Verification items for the finished model (mm, model axes). Face numbers are marked on the shaded views. A direction names the side the tool comes from. Round coordinates to 2 decimals unless told otherwise and drop trailing zeros. Write each loop counter-clockwise with the first axis right and the second up, starting at its lowest first coordinate (ties: lowest second). Pieces come first, ordered by that corner, then holes.
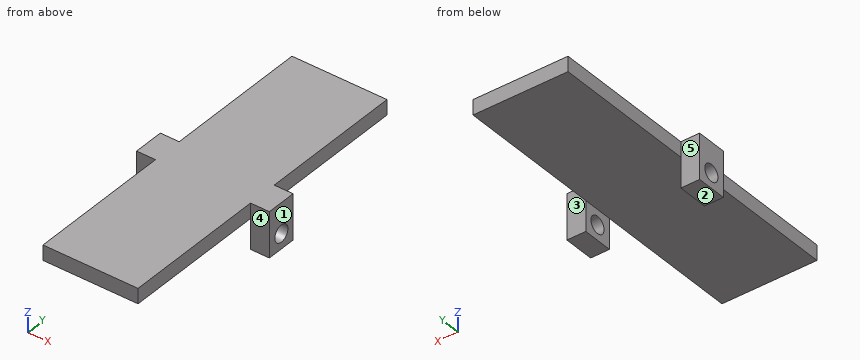
from build123d import *

# Parameters (mm, degrees)
SKETCH1_W           = 16
SKETCH1_H           = 54.011330832
BOSS_EXTRUDE1_DEPTH = 2.54
SKETCH2_W           = 7.62
SKETCH2_H           = 5.141453329
SKETCH2_R           = 1.4224
BOSS_EXTRUDE2_DEPTH = 3.175


with BuildPart() as part:
    # Sketch1 → Boss-Extrude1 (new body)
    with BuildSketch(Plane.XY):
        with Locations((-8, 27.005665416)):
            Rectangle(SKETCH1_W, SKETCH1_H)
    extrude(amount=BOSS_EXTRUDE1_DEPTH)

    # Sketch2 → Boss-Extrude2 (add)
    with BuildSketch(Plane(origin=(0, 0, 0), x_dir=(0, 0, -1), z_dir=(1, 0, 0))):
        with Locations((1.27, 26.974938752)):
            Rectangle(SKETCH2_W, SKETCH2_H)
        with Locations((2.54, 27.005665416)):
            Circle(SKETCH2_R, mode=Mode.SUBTRACT)
    boss_extrude2 = extrude(amount=BOSS_EXTRUDE2_DEPTH)

    # Mirror1: Boss-Extrude2 across plane
    add(boss_extrude2.mirror(Plane.ZY.offset(8)))


solid = part.part
Q1. Sectioned sample at A-A (z = -2.54). Enter the section's corners in (x, y) (3 decimals), plus the area to 3 significant figures.
Recorded:
outline: (-19.175, 24.404) - (-16, 24.404) - (-16, 25.583) - (-19.175, 25.583) - close; (-19.175, 28.428) - (-16, 28.428) - (-16, 29.546) - (-19.175, 29.546) - close; (0, 24.404) - (3.175, 24.404) - (3.175, 25.583) - (0, 25.583) - close; (0, 28.428) - (3.175, 28.428) - (3.175, 29.546) - (0, 29.546) - close
area: 14.6 mm2
Q2. Sectioned sample at C-C (x = -17.5). Enter the section's corners in (y, z), plus the area to 3 significant figures.
Recorded:
outline: (24.4, -5.08) - (29.55, -5.08) - (29.55, 2.54) - (24.4, 2.54) - close; hole circle Ø2.84 at (27.01, -2.54)
area: 32.8 mm2
Q3. Depth check by flat-ended pin: P1, Ø1, axis at x = 1, z = -1.5, coming from the -Y side; P2, Ø3, axis at y = 19, z = -1, coming from the +X side; P3, Ø2.5, axis at x = -18, z = 0, coming from the +Y side; P4, Ø2, axis at y = 44.5, z = -1.5, coming from the -X side. Enter the tip coordinate at first touch or a pass-through.
Recorded:
P1: stops at y = 24.4
P2: stops at x = 0
P3: stops at y = 29.55
P4: passes through
Q4. Sectioned sample at B-B (z = 1.5). Enter the section's corners in (x, y) (3 decimals), plus the area to 3 significant figures.
Recorded:
outline: (-19.175, 24.404) - (-16, 24.404) - (-16, 0) - (0, 0) - (0, 24.404) - (3.175, 24.404) - (3.175, 29.546) - (0, 29.546) - (0, 54.011) - (-16, 54.011) - (-16, 29.546) - (-19.175, 29.546) - close
area: 897 mm2
Q5. Sectioned sample at D-D (y = 42). Enter the section's corners in (x, z).
Recorded:
outline: (-16, 0) - (0, 0) - (0, 2.54) - (-16, 2.54) - close
Q6. Material ranges on line 1 along Y through (x, z) = (-17.3, -2.54); line 2 along X through (y, z) = (24.5, -1) (3 decimals); line 3 along Y through (x, z) = (-17, 2), recorded low to high.
Recorded:
line 1: y = 24.4 to 25.58, 28.43 to 29.55
line 2: x = -19.175 to -16, 0 to 3.175
line 3: y = 24.4 to 29.55
Q7. Tool access check on the marked faces 1, 2, 3, 4 and 5. Record the directions out of +Z, -Z, +X, -X, +Y, -Y that give a thin tool (end or side, any length) a straight path to the whole face; none if there is none.
Recorded:
face 1: +Z, -Z, +X, +Y, -Y
face 2: -Z, +X, -X, +Y, -Y
face 3: +Z, -Z, +X, +Y
face 4: +Z, -Z, +X, -Y
face 5: +Z, -Z, -X, +Y
